The listing builds one solid part. Answer for the finished solid, in the listing's coordinates (mm). A direction names the side the tool comes from. Round coordinates to 2 decimals unless told otherwise and drop trailing zeros. Loops run counter-clockwise (first coordinate to the right, second up) from the corner with the lowest first, then second, coordinate; pieces in that order, holes last. Notation, with made-up numbers: M 12.5,41 L 40.5,41 A24 ccw 40.5,68 Z; hole C -18.75,5.25 d3. An arc over 180 degrees is marked long. Put each result on its own line as item: value. Start each with the question number.
(1) Section C-C, the plane y = -8 is taken. Determine the outline of the cut face in (x, z), then the cut area to 3 significant figures.
(2) Section B-B, the plane z = 0.6 is taken. Determine the outline of the cut face in (x, y), then the cut area to 3 significant figures.
(3) Section D-D, the plane z = 3.55 is taken. Determine the outline of the cut face in (x, y).
(4) Flat-ended cylindrical pins translate along their axes: P1, Ø1.9, axis at x = 0.5, y = 0, coming from the -Z side; P2, Ø2.5, axis at x = 1.5, y = -4.5, coming from the +Z side; P3, Ø0.7, axis at x = -0.5, y = 7.5, coming from the -Z side. Find the tip coordinate at first contact, or state that the pin passes through.
(5) Straight lines are drawn through the part: line 1 (Y direction, x = 0, z = 2.25); line 2 (Y direction, x = -0.75, z = 3.65); line 3 (X direction, y = 9, z = 0.45). For each, find the intervals that lie inside material, in ascending order.
(6) Which of the six approach directions +Z, -Z, +X, -X, +Y, -Y give full straight-line access (tool end or side, diameter ignored) to faces 5 (the face through (0, 3, 3.2)), 6 (the face through (0, 8, 4.8)), 7 (the face through (-0.65, 9.01, 2.49))?
(7) Determine the mould class of faces 1 (the face through (0, -12, 2)), 2 (the face through (0, 12, 2)), 3 (the face through (-3, 0, 0)), 4 (the face through (-0.65, -6.99, 2.49)) for opening direction Y: released by +Y, released by -Y, zero draft, split by the parting line, or undercut.
Autodesk Inventor part; units mm, degrees
ref_plane "YZ Plane" through (0, 0, 0) normal (1, 0, 0) x (0, 1, 0)
ref_plane "XZ Plane" through (0, 0, 0) normal (0, 1, 0) x (-1, 0, 0)
ref_plane "XY Plane" through (0, 0, 0) normal (0, 0, 1) x (1, 0, 0)
sketch "Sketch1" plane through (0, 0, 0) normal (0, 0, 1) x (1, 0, 0)
  line L0 (-4, 12) -> (4, 12)
  line L1 (4, 12) -> (4, -12)
  line L2 (4, -12) -> (-4, -12)
  line L3 (-4, -12) -> (-4, 12)
  point P0 (0, 0)
  dimension "d0" = 8
  dimension "d1" = 24
  dimension "d2" = 4
  dimension "d3" = 12
extrude "Extrusion1" add sketch "Sketch1" along normal blind 3.2
shell "Shell1" thickness 1.5 removed faces 1 at (-1.3333, 4, 0)
sketch "Sketch2" plane through (0, 0, 3.2) normal (0, 0, 1) x (1, 0, 0)
  circle A0 centre (0, -8) radius 2.5
  line L0 (4, 12) -> (4, -12)
  line L1 (4, -12) -> (-4, -12)
  dimension "d7" = 5
  dimension "d10" = 4
  dimension "d11" = 4
extrude "Extrusion2" add sketch "Sketch2" along normal blind 1.6
sketch "Sketch3" plane through (2.5, -10.5, 1.7) normal (0, 0, -1) x (-1, 0, 0)
  circle A0 centre (2.5, 2.5) radius 2.5
  circle A1 centre (2.5, 2.5) radius 1.2
  point P0 (2.5, 10.5)
  dimension "d18" = 2.4
extrude "Extrusion3" cut sketch "Sketch3" against normal blind 1.6 contours A1
pattern_linear "Rectangular Pattern1" count 3 spacing 8 along (0, 1, 0) of "Extrusion2", "Extrusion3"
sketch "Sketch4" plane through (2.5, -10.5, 1.7) normal (0, 0, -1) x (-1, 0, 0)
  circle A0 centre (2.5, 10.5) radius 1.2
  circle A1 centre (2.5, 2.5) radius 1.2
  line L0 (0, 21) -> (0, 0)
  line L1 (0, 0) -> (5, 0)
  circle A2 centre (6.5, 6.5) radius 3.15
  circle A3 centre (6.5, 6.5) radius 2.5
  point P0 (2.5, 10.5)
  dimension "d21" = 6.5
  dimension "d22" = 6.5
  dimension "d23" = 10.5
  dimension "d24" = 2.5
  dimension "d25" = 5
  dimension "d26" = 6.3
extrude "Extrusion4" [suppressed]
pattern_linear "Rectangular Pattern2" [suppressed]
equation "\"d0\" = 0.8 * WIDTH"
equation "\"d1\" = 0.8 * LENGTH"
equation "\"d4\" = HEIGHT"
equation "\"d21\" = 0.5 * d23 + 0.5 * d24"
equation "\"d22\" = d21"
equation "\"WIDTH\" = 1"
equation "\"HEIGHT\" = 3.2"
properties part number "3623" material "Steel"
Recorded:
1. outline: M -4,0 L -2.5,0 L -2.5,1.7 L -1.2,1.7 L -1.2,3.3 L 1.2,3.3 L 1.2,1.7 L 2.5,1.7 L 2.5,0 L 4,0 L 4,3.2 L 2.5,3.2 L 2.5,4.8 L -2.5,4.8 L -2.5,3.2 L -4,3.2 Z
1. area: 21.3 mm²
2. outline: M -4,-12 L 4,-12 L 4,12 L -4,12 Z; hole M -2.5,-10.5 L 2.5,-10.5 L 2.5,10.5 L -2.5,10.5 Z
2. area: 87.0 mm²
3. outline: C 0,-8 d5; C 0,0 d5; C 0,8 d5
4. P1: stops at z = 1.7
4. P2: stops at z = 3.2
4. P3: stops at z = 3.3
5. line 1: y = -12 to -9.2, -6.8 to -1.2, 1.2 to 6.8, 9.2 to 12
5. line 2: y = -10.38 to -5.62, -2.38 to 2.38, 5.62 to 10.38
5. line 3: x = -4 to -2.5, 2.5 to 4
6. face 5: +Z
6. face 6: +Z, +X, -X, +Y, -Y
6. face 7: -Z
7. face 1: released by -Y
7. face 2: released by +Y
7. face 3: zero draft
7. face 4: undercut
